```python
from build123d import *

# Parameters (mm, degrees)
SKETCH_3_R           = 5
SKETCH_4_R           = 5
SKETCH_2_R           = 5
SKETCH_7_R           = 5
SKETCH_7_R_2         = 1.45
CUT_EXTRUDE_1_DEPTH  = 12
SKETCH_8_R           = 5
SKETCH_8_R_2         = 1.45
CUT_EXTRUDE_2_DEPTH  = 12
SKETCH_9_R           = 5
SKETCH_9_R_2         = 1.45
CUT_EXTRUDE_3_DEPTH  = 12
EXTRUDE_1_DEPTH      = 40
EXTRUDE_1_DEPTH_BACK = 60
SKETCH_10_R          = 5
SKETCH_12_R          = 5
SKETCH_12_R_2        = 1.45
CUT_EXTRUDE_5_DEPTH  = 12


with BuildPart() as part:
    # 扫描1: sweep along a path in 草图1
    with BuildLine(Plane(origin=(0, 0, 0), x_dir=(1, 0, 0), z_dir=(0, 1, 0))) as sweep_1_path:
        Line((0, 0), (53.333333333, -20))
    # 草图3 → 扫描1 (sweep)
    with BuildSketch(Plane(origin=(0, 0, 0), x_dir=(0.35112344158838826, 0, -0.9363291775690458), z_dir=(0.9363291775690458, 0, 0.35112344158838826))):
        Circle(SKETCH_3_R)
    sweep(path=sweep_1_path.line)

    # 扫描7: sweep along a path in 草图5
    with BuildLine(Plane(origin=(0, 0, 0), x_dir=(1, 0, 0), z_dir=(0, 1, 0))) as sweep_7_path:
        Line((0, 0), (-26.666666667, 40))
    # 草图4 → 扫描7 (sweep)
    with BuildSketch(Plane(origin=(0, 0, 0), x_dir=(0.8320502943378456, 0, -0.5547001962252264), z_dir=(0.5547001962252264, 0, 0.8320502943378456))):
        Circle(SKETCH_4_R)
    sweep(path=sweep_7_path.line)

    # 扫描8: sweep along a path in 草图6
    with BuildLine(Plane(origin=(0, 0, 0), x_dir=(1, 0, 0), z_dir=(0, 1, 0))) as sweep_8_path:
        Line((0, 0), (-26.666666667, -20))
    # 草图2 → 扫描8 (sweep)
    with BuildSketch(Plane(origin=(0, 0, 0), x_dir=(0.600000000000003, 0, 0.7999999999999979), z_dir=(-0.7999999999999979, 0, 0.600000000000003))):
        Circle(SKETCH_2_R)
    sweep(path=sweep_8_path.line)

    # 草图7 → 切除-拉伸1 (cut)
    with BuildSketch(Plane(origin=(-26.666666667, 0, -40), x_dir=(-0.8320502943378455, 0, 0.5547001962252265), z_dir=(-0.5547001962252265, 0, -0.8320502943378456))):
        Circle(SKETCH_7_R)
        Circle(SKETCH_7_R_2, mode=Mode.SUBTRACT)
    extrude(amount=-CUT_EXTRUDE_1_DEPTH, mode=Mode.SUBTRACT)

    # 草图8 → 切除-拉伸2 (cut)
    with BuildSketch(Plane(origin=(-26.666666667, 0, 20), x_dir=(0.6000000000000031, 0, 0.7999999999999977), z_dir=(-0.7999999999999977, 0, 0.6000000000000031))):
        Circle(SKETCH_8_R)
        Circle(SKETCH_8_R_2, mode=Mode.SUBTRACT)
    extrude(amount=-CUT_EXTRUDE_2_DEPTH, mode=Mode.SUBTRACT)

    # 草图9 → 切除-拉伸3 (cut)
    with BuildSketch(Plane(origin=(53.333333333, 0, 20), x_dir=(0.35112344158838826, 0, -0.9363291775690458), z_dir=(0.9363291775690458, 0, 0.35112344158838826))):
        Circle(SKETCH_9_R)
        Circle(SKETCH_9_R_2, mode=Mode.SUBTRACT)
    extrude(amount=-CUT_EXTRUDE_3_DEPTH, mode=Mode.SUBTRACT)

    # 草图10 → 凸台-拉伸1 (add, two sides: drawn at the far end of the back side and taken through both)
    with BuildSketch(Plane(origin=(0, 0, 0), x_dir=(1, 0, 0), z_dir=(0, 1, 0)).offset(-EXTRUDE_1_DEPTH_BACK)):
        with Locations(Location((0, 0, 0), (0, 0, 270))):
            Circle(SKETCH_10_R)
    extrude(amount=EXTRUDE_1_DEPTH + EXTRUDE_1_DEPTH_BACK)

    # 草图12 → 切除-拉伸5 (cut)
    with BuildSketch(Plane(origin=(0, 40, 0), x_dir=(1, 0, 0), z_dir=(0, 1, 0))):
        with Locations(Location((0, 0, 0), (0, 0, 270))):
            Circle(SKETCH_12_R)
        with Locations(Location((0, 0, 0), (0, 0, 270))):
            Circle(SKETCH_12_R_2, mode=Mode.SUBTRACT)
    extrude(amount=-CUT_EXTRUDE_5_DEPTH, mode=Mode.SUBTRACT)

    # 草图13 → 切除-旋转1 (revolve, cut)
    with BuildSketch(Plane(origin=(0, 0, 0), x_dir=(0, 0, -1), z_dir=(1, 0, 0))):
        with BuildLine():
            Line((-1, -59.017604387), (-1, -20.025015645))
            ThreePointArc((-1, -20.025015645), (-19.897410745, -37.976872316), (-5, -59.364916731))
            Line((-5, -59.364916731), (-5, -59.017604387))
            Line((-5, -59.017604387), (-1, -59.017604387))
        make_face()
        with BuildLine():
            Line((-1, -59.974984355), (-1, -59.017604387))
            Line((-1, -59.017604387), (-5, -59.017604387))
            Line((-5, -59.017604387), (-5, -59.364916731))
            ThreePointArc((-5, -59.364916731), (-3.015467729, -59.771367034), (-1, -59.974984355))
        make_face()
        with BuildLine():
            ThreePointArc((-1, -59.974984355), (-3.015467729, -59.771367034), (-5, -59.364916731))
            Line((-5, -59.364916731), (-5, -60))
            Line((-5, -60), (-1, -60))
            Line((-1, -60), (-1, -59.974984355))
        make_face()
    revolve(axis=Axis((0, -1000, 0), (0, 1, 0)), mode=Mode.SUBTRACT)


solid = part.part
```
CAD build for the part. Positions are in the model's coordinates, mm. A direction names the side the tool comes from. Round coordinates to 2 decimals unless told otherwise and drop trailing zeros. Write each loop counter-clockwise with the first axis right and the second up, starting at its lowest first coordinate (ties: lowest second). Pieces come first, ordered by that corner, then holes. Notation, with made-up numbers: (-10, 23.25) - (4, 23.25) arc R28 ccw to (4, 57.25) - close; hole circle Ø4 at (26, 45.25). An arc over 180 degrees is marked (long way). Return JSON: item names as keys, results as strings. Group by question number.
Item 1: Flat gauge pins, fed straight in: pin 1 Ø12 at (x, y) = (6, -25.5) entering from +Z; pin 2 Ø2 at (x, y) = (1.5, -40.5) entering from -Z; pin 3 Ø6 at (y, z) = (12, 7.5) entering from +X. Where does each tip first touch, or does it go through?
Item 2: 3-axis set-ups, long thin cutter, end or side, ignore diameter. For faces 1 (the face through (41.683, 1.181, 16.892)), 2 (the face through (3, 15, -4)), 3 (the face through (53.34, -0.02, 19.98)), 4 (the face through (3, -13, -4)), 5 (the face through (0, 40, 0)): which of +Z, -Z, +X, -X, +Y, -Y reach the whole face in a straight line?
Item 3: Mould opens along Z. For faces 6 (the face through (-26.65, -0.02, 20.02)), 7 (the face through (21.823, 4.957, 8.879)), 8 (the face through (-22.18, 0.06, -35.88)), 9 (the face through (1.2, 28, -1.2)) say: +Z half, -Z half, draft (parallel to the pull), parting line (faces both ways), or undercut.
Item 4: Band-saw the part on A-A on y = 18. List the corners of the cut face in (x, z), plus the area to 3 significant figures.
Item 5: Probe probe 1 along Y at (x, z) = (-17.5, -27); probe 2 along X at (y, z) = (-4.5, -29); probe 3 along Z at (x, y) = (30.5, -2.5). List the from-to ranges inside material, lowest first.
Resolved:
{
 "1": {"pin 1": "stops at z = 4.34", "pin 2": "stops at z = -0.87", "pin 3": "stops at x = 2.18"},
 "2": {"face 1": "none", "face 2": "+Y", "face 3": "+Z, +X, +Y, -Y", "face 4": "-Y", "face 5": "+Z, -Z, +X, -X, +Y"},
 "3": {"face 6": "+Z half", "face 7": "parting line", "face 8": "undercut", "face 9": "draft"},
 "4": {"outline": "circle Ø10 at (0, 0)", "area": "78.5 mm²"},
 "5": {"probe 1": "y = -4.98 to 4.98", "probe 2": "x = -21.53 to -16.71", "probe 3": "z = 6.81 to 16.06"}
}
